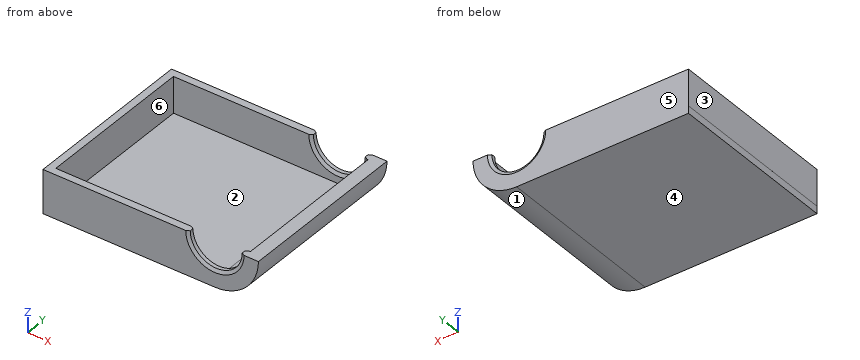
```python
from build123d import *

# Parameters (mm, degrees)
PAD005_DEPTH        = 70.75
PAD006_DEPTH        = 14.75
PAD007_DEPTH        = 3
PAD008_DEPTH        = 3
POCKET001_DEPTH     = 70.751
REVOLUTION001_ANGLE = 180
SKETCH013_W         = 2.5
SKETCH013_H         = 8.75
PAD009_DEPTH        = 67.75


with BuildPart() as part:
    # Sketch007 → Pad005 (new body)
    with BuildSketch(Plane.XZ):
        with BuildLine():
            ThreePointArc((0, 0), (10.429825, 4.320175), (14.75, 14.75))
            Line((14.75, 14.75), (17.75, 14.75))
            ThreePointArc((4.3e-05, -3), (12.55116, 2.19887), (17.75, 14.75))
            Line((-69.999957, -3), (4.3e-05, -3))
            Line((-69.999957, 0), (-69.999957, -3))
            Line((0, 0), (-69.999957, 0))
        make_face()
    extrude(amount=PAD005_DEPTH)

    # Sketch008 (on Face6 of Pad005) → Pad006 (join)
    with BuildSketch(Plane(origin=(0, 0, 0), x_dir=(-1, 0, 0), z_dir=(0, 0, 1))):
        Polygon((70, 0), (70, 70.75), (0, 70.75), (0, 67.75), (67, 67.75), (67, 3), (0, 3), (0, 0), align=None)
    extrude(amount=PAD006_DEPTH)

    # Sketch009 (on Face15 of Pad006) → Pad007 (join)
    with BuildSketch(Plane.XZ.offset(70.75)):
        with BuildLine():
            ThreePointArc((0, 0), (10.429825, 4.320175), (14.75, 14.75))
            Line((0, 14.75), (14.75, 14.75))
            Line((0, 0), (0, 14.75))
        make_face()
    extrude(amount=-PAD007_DEPTH)

    # Sketch010 (on Face2 of Pad007) → Pad008 (join)
    with BuildSketch(Plane(origin=(0, 0, 0), x_dir=(1, 0, 0), z_dir=(0, 1, 0))):
        with BuildLine():
            ThreePointArc((14.75, -14.75), (10.429825, -4.320175), (0, 0))
            Line((0, -14.75), (0, 0))
            Line((14.75, -14.75), (0, -14.75))
        make_face()
    extrude(amount=-PAD008_DEPTH)

    # Sketch011 (on Face2 of Pad008) → Pocket001 (cut, through all)
    with BuildSketch(Plane.XZ.offset(70.75)):
        with BuildLine():
            ThreePointArc((-11.875, 14.75), (0, 2.875), (11.875, 14.75))
            Line((-11.875, 14.75), (11.875, 14.75))
        make_face()
    extrude(amount=-POCKET001_DEPTH, mode=Mode.SUBTRACT)

    # Sketch012 (on Face5 of Pocket001) → Revolution001 (revolve)
    with BuildSketch(Plane(origin=(0, 0, 14.75), x_dir=(-1, 0, 0), z_dir=(0, 0, 1))):
        Polygon((13.174038, 70), (11.875, 70.75), (10.575962, 70), (10.575962, 68.5), (11.875, 67.75), (13.174038, 68.5), align=None)
        Polygon((13.174038, 2.25), (11.875, 3), (10.575962, 2.25), (10.575962, 0.75), (11.875, 0), (13.174038, 0.75), align=None)
    revolve(axis=Axis((0, 0, 14.75), (0, -1, 0)), revolution_arc=REVOLUTION001_ANGLE)

    # Sketch013 (on Face3 of Revolution001) → Pad009 (join)
    with BuildSketch(Plane(origin=(0, -67.75, 0), x_dir=(1, 0, 0), z_dir=(0, 1, 0))):
        with Locations((13.5, -10.375)):
            Rectangle(SKETCH013_W, SKETCH013_H)
    extrude(amount=PAD009_DEPTH)


solid = part.part
```
Geometry: final body of the model. Coordinates: model frame, mm. Face numbers are marked on the shaded views. A direction names the side the tool comes from. Coordinates: 2 decimals unless noted, no trailing zeros. Order: outer loops, then holes, each group sorted by start corner. A loop starts at its lowest first (then second) coordinate and runs counter-clockwise, first axis right, second up.
Item 1: Section query C-C (z = -1.5). Output: boundary loops of the cut face in (x, y), then the cut area to 3 significant figures.
Answer:
outline: (-70, -70.75) - (7.14, -70.75) - (7.14, 0) - (-70, 0) - close
area: 5,460 mm2
Item 2: Access query for the marked faces 5 and 6. Directions: +Z, -Z, +X, -X, +Y, -Y. A direction counts if a zero-diameter tool reaches every point of the face in a straight line with its end or side. Return the directions, or none.
Answer:
face 5: +Z, -Z, +X, -X, +Y
face 6: +Z
Item 3: Draft query along X for the marked faces 1, 2, 3 and 4. Return one class per face: released by +X, released by -X, zero draft, split by the parting line, or undercut.
Answer:
face 1: released by +X
face 2: undercut
face 3: released by -X
face 4: zero draft
Item 4: Material intervals for line 1 along Y through (x, z) = (-20.5, 4.5); line 2 along Z through (x, y) = (-12.5, -12); line 3 along X through (y, z) = (-9, 7.75), sorted ascending.
Answer:
line 1: y = -70.75 to -67.75, -3 to 0
line 2: z = -3 to 0
line 3: x = -70 to -67, 12.25 to 16.31
Item 5: Contact query for flat-ended pins moving along their axis: P1, Ø6, axis at y = -15, z = 10.5, coming from the +X side; P2, Ø4.5, axis at y = -39, z = 6, coming from the +X side; P3, Ø19.5, axis at x = -34.5, y = -36, coming from the +Z side. Output: stop coordinate, or through.
Answer:
P1: stops at x = 17.71
P2: stops at x = 16.52
P3: stops at z = 0
Item 6: Section query B-B (x = -44.5). Output: boundary loops of the cut face in (y, z).
Answer:
outline: (-70.75, -3) - (0, -3) - (0, 14.75) - (-3, 14.75) - (-3, 0) - (-67.75, 0) - (-67.75, 14.75) - (-70.75, 14.75) - close
